Could you check a few things on this model? Use its own coordinates, in mm. A direction names the side the tool comes from. Coordinates: 2 decimals unless noted, no trailing zeros. Write item = value, one per line.
Autodesk Inventor part; units mm, degrees
ref_plane "YZ Plane" through (0, 0, 0) normal (1, 0, 0) x (0, 1, 0)
ref_plane "XZ Plane" through (0, 0, 0) normal (0, 1, 0) x (-1, 0, 0)
ref_plane "XY Plane" through (0, 0, 0) normal (0, 0, 1) x (1, 0, 0)
sketch "Sketch1" plane through (0, 0, 0) normal (0, 0, 1) x (1, 0, 0)
  circle A0 centre (4.9, 14.6) radius 0.455
  circle A1 centre (4.9, 14.6) radius 0.7
  line L0 (6.3, 13.375) -> (6.3, 14.6)
  line L1 (0, 26) -> (7, 26)
  line L2 (7, 26) -> (7, 24.75)
  line L3 (7, 24.75) -> (1.75, 24.75)
  line L4 (0, 0) -> (9.5856, 0)
  line L5 (0, 26) -> (0, 14.6)
  line L6 (0, 14.6) -> (1.75, 14.25)
  line L7 (1.75, 14.25) -> (4.9, 12.5)
  line L8 (4.9, 12.5) -> (6.3, 13.375)
  line L9 (4.9, 12.5) -> (0, 12.5) construction
  line L10 (0, 18) -> (0, -3)
  line L11 (-1.9171, 0) -> (11.5027, 0)
  line L12 (4.2, 14.6) -> (1.75, 15.09)
  line L13 (1.75, 15.09) -> (1.75, 24.75)
  line L14 (6.3, 14.6) -> (5.6, 14.6)
  dimension "d0" = 52
  dimension "d1" = 26.75
  dimension "d2" = 1.25
  dimension "d3" = 0.91
  dimension "d4" = 1.4
  dimension "d5" = 25
  dimension "d6" = 28.5
  dimension "d7" = 29.2
  dimension "d8" = 4.9
  dimension "d9" = 6.3
  dimension "d10" = 7
  dimension "d12" = 1.75
revolve "Body" add sketch "Sketch1" angle 360 about axis through (0, 0, 0) along (1, 0, 0) contours L14 L0 L8 L7 L6 L5 L1 L2 L3 L13 L12 A1
revolve "Spring1" add sketch "Sketch1" angle 360 about axis through (0, 0, 0) along (1, 0, 0) contours A0 | A1
fillet "Fillet1" radius 0.3 3 edges at (7, -26, 0) (1.75, -24.75, 0) (0, -26, 0)
equation "\"d0\" = SD2"
equation "\"d1\" = ABDM"
equation "\"d3\" = SPDI"
equation "\"d4\" = SPDA"
equation "\"d5\" = NND"
equation "\"d6\" = TKDM"
equation "\"d7\" = HLDM"
equation "\"d8\" = SPDST"
equation "\"d9\" = SDI"
equation "\"d10\" = SWDT"
equation "\"d12\" = SD"
equation "\"d11\" = RR"
equation "\"SD2\" = 52"
equation "\"SWDT\" = 7"
equation "\"RR\" = 0.3"
equation "\"SD\" = 1.75"
equation "\"NND\" = 25"
equation "\"SPDA\" = 1.4"
equation "\"SPDI\" = 0.91"
equation "\"TKDM\" = 28.5"
equation "\"HLDM\" = 29.2"
equation "\"ABDM\" = 26.75"
equation "\"SDI\" = 6.3"
equation "\"SPDST\" = 4.9"
equation "\"LAB\" = 0.35"
properties part number "CSN 02 9401 - G 25x52x7 - NBR" material "Rubber"
Item 1: For faces 1 (the face through (6.3, 13, -4)), 2 (the face through (4.047, 13.955, -4.395)), 3 (the face through (0, 11, -11)), which set-ups out of +Z, -Z, +X, -X, +Y, -Y let a thin tool reach every point of the face, with its end or its side?
Numbers:
face_1 = +X
face_2 = none
face_3 = +Z, -Z, -X, +Y, -Y
Item 2: If I drill on line 1 along Z through (x, y) = (6, 1); line 2 along Z through (x, y) = (2.25, -12); line 3 along Y through (x, z) = (3.5, -7), over which ranges is the centre line in solid material (lowest first)?
Numbers:
line_1 = -25.98 to -24.73, -14.57 to -13.15, 13.15 to 14.57, 24.73 to 25.98
line_2 = -23.07 to -21.65, -8.98 to -7.16, 7.16 to 8.98, 21.65 to 23.07
line_3 = -25.04 to -23.74, -12.97 to -11.28, 11.28 to 12.97, 23.74 to 25.04
Item 3: I'm going to push flat-ended pins straight in: P1, Ø8, axis at y = -9, z = 8.5, coming from the +X side; P2, Ø4, axis at x = 1.5, z = 9.5, coming from the +Y side; P3, Ø3, axis at x = 2.5, y = 7.5, coming from the +Z side. Where does each tip first touch, or does it pass through?
Numbers:
P1 = 6.3
P2 = 24.89
P3 = 25.3
Item 4: If we mould it in two halves opening along Y, with no side actions, what happens to faces 4 (the face through (1.75, -11, -11)), 5 (the face through (3.545, -20.633, -15.821)), 6 (the face through (7, -13.4, 21.1))? For each: pulls with the +Y half, pulls with the -Y half, needs draft (parallel to the pull), parting line crosses it, or undercut.
Numbers:
face_4 = undercut
face_5 = parting line crosses it
face_6 = needs draft
